Here's how the part is built. I have some questions about the finished solid (model axes, mm). A direction names the side the tool comes from. Give positions to 0.01 mm unless a question says otherwise; leave off trailing zeros. Write each loop counter-clockwise with the first axis right and the second up, starting at its lowest first coordinate (ties: lowest second). Pieces come first, ordered by that corner, then holes. Notation, with made-up numbers: (20, 5) -> (43, 5) arc R19 cw to (43, 13) -> close; hole circle Ø9 at (-12, -23). An arc over 180 degrees is marked (long way). Put each result on its own line as item: value. Start each with the question number.
from build123d import *

# Parameters (mm, degrees)
SKETCH1_W                    = 288.2
SKETCH1_H                    = 200
SKETCH1_R                    = 5
BASE_FLANGE1_DEPTH           = 3.4
EDGE_FLANGE2_STRIP_W         = 15.0732
EDGE_FLANGE2_STRIP_H         = 3.4
EDGE_FLANGE2_STRIP_CUT_DEPTH = 200
EDGE_FLANGE2_DEPTH           = 200
EDGE_FLANGE2_PROFILE_W       = 200
EDGE_FLANGE2_PROFILE_H       = 39.2634
EDGE_FLANGE2_PROFILE_R       = 5
EDGE_FLANGE2_FLAT_DEPTH      = 3.4
EDGE_FLANGE3_STRIP_W         = 15.0732
EDGE_FLANGE3_STRIP_H         = 3.4
EDGE_FLANGE3_STRIP_CUT_DEPTH = 200
EDGE_FLANGE3_DEPTH           = 200
EDGE_FLANGE3_PROFILE_W       = 200
EDGE_FLANGE3_PROFILE_H       = 39.2634
EDGE_FLANGE3_PROFILE_R       = 5
EDGE_FLANGE3_FLAT_DEPTH      = 3.4


# Sheet-metal steps are written as plain solids
with BuildPart() as part:
    # Sketch1 → Base-Flange1 (new body)
    with BuildSketch(Plane.XY):
        with Locations((-144.1, -100)):
            Rectangle(SKETCH1_W, SKETCH1_H)
        with Locations((-111.6, -100)):
            Circle(SKETCH1_R, mode=Mode.SUBTRACT)
        with Locations(Location((-176.6, -100, 0), (0, 0, 180))):
            Circle(SKETCH1_R, mode=Mode.SUBTRACT)
    extrude(amount=-BASE_FLANGE1_DEPTH)

    # Edge-Flange2 strip (across the edge) → Edge-Flange2 strip cut (cut)
    with BuildSketch(Plane(origin=(0, 0, -3.4), x_dir=(-1, 0, 0), z_dir=(0, -1, 0))):
        with Locations((-3.4, -1.7)):
            Rectangle(EDGE_FLANGE2_STRIP_W, EDGE_FLANGE2_STRIP_H)
    extrude(amount=EDGE_FLANGE2_STRIP_CUT_DEPTH, mode=Mode.SUBTRACT)

    # Edge-Flange2 bend section (across the edge) → Edge-Flange2 (add)
    with BuildSketch(Plane(origin=(0, 0, -3.4), x_dir=(-1, 0, 0), z_dir=(0, -1, 0))):
        with BuildLine():
            Line((0, 0.7366), (3.4, 0.7366))
            ThreePointArc((3.4, 0.7366), (3.615745145, 0.215745145), (4.1366, 0))
            Line((4.1366, 0), (4.1366, -3.4))
            ThreePointArc((4.1366, -3.4), (1.211582089, -2.188417911), (0, 0.7366))
        make_face()
    extrude(amount=EDGE_FLANGE2_DEPTH)

    # Edge-Flange2 profile (on flange) → Edge-Flange2 flat (add)
    with BuildSketch(Plane(origin=(0, 0, -3.4), x_dir=(0, -1, 0), z_dir=(1, 0, 0))):
        with Locations((100, 20.3683)):
            Rectangle(EDGE_FLANGE2_PROFILE_W, EDGE_FLANGE2_PROFILE_H)
        with Locations((150, 15.6)):
            Circle(EDGE_FLANGE2_PROFILE_R, mode=Mode.SUBTRACT)
        with Locations((50, 15.6)):
            Circle(EDGE_FLANGE2_PROFILE_R, mode=Mode.SUBTRACT)
    extrude(amount=-EDGE_FLANGE2_FLAT_DEPTH)

    # Edge-Flange3 strip (across the edge) → Edge-Flange3 strip cut (cut)
    with BuildSketch(Plane(origin=(-288.2, -200, -3.4), x_dir=(1, 0, 0), z_dir=(0, 1, 0))):
        with Locations((-3.4, -1.7)):
            Rectangle(EDGE_FLANGE3_STRIP_W, EDGE_FLANGE3_STRIP_H)
    extrude(amount=EDGE_FLANGE3_STRIP_CUT_DEPTH, mode=Mode.SUBTRACT)

    # Edge-Flange3 bend section (across the edge) → Edge-Flange3 (add)
    with BuildSketch(Plane(origin=(-288.2, -200, -3.4), x_dir=(1, 0, 0), z_dir=(0, 1, 0))):
        with BuildLine():
            Line((0, 0.7366), (3.4, 0.7366))
            ThreePointArc((3.4, 0.7366), (3.615745145, 0.215745145), (4.1366, 0))
            Line((4.1366, 0), (4.1366, -3.4))
            ThreePointArc((4.1366, -3.4), (1.211582089, -2.188417911), (0, 0.7366))
        make_face()
    extrude(amount=EDGE_FLANGE3_DEPTH)

    # Edge-Flange3 profile (on flange) → Edge-Flange3 flat (add)
    with BuildSketch(Plane(origin=(-288.2, 0, -3.4), x_dir=(0, 1, 0), z_dir=(-1, 0, 0))):
        with Locations((-100, 20.3683)):
            Rectangle(EDGE_FLANGE3_PROFILE_W, EDGE_FLANGE3_PROFILE_H)
        with Locations((-50, 15.6)):
            Circle(EDGE_FLANGE3_PROFILE_R, mode=Mode.SUBTRACT)
        with Locations((-150, 15.6)):
            Circle(EDGE_FLANGE3_PROFILE_R, mode=Mode.SUBTRACT)
    extrude(amount=-EDGE_FLANGE3_FLAT_DEPTH)


solid = part.part
1) I need wall thicknesses on probe 1 along Y at (x, z) = (-285.95, -19); probe 2 along X at (y, z) = (-117.5, -15.5); probe 3 along Y at (x, z) = (-176.6, -1). Which ranges of each line are inside material? Lowest first, please.
2) I'm going to push a flat-ended pin straight in: pin 1 Ø10 at (x, y) = (-114.5, -174) entering from -Z. Where does the tip first touch, or does it pass through?
3) Which directions (+Z, -Z, +X, -X, +Y, -Y) give clear straight access to the entire face, cutting with the end or side of a thin tool? Please do faces 5 (the flat face through (-145, -200, -1)), 6 (the flat face through (-3.4, -99, -24)).
4) I want a section at A-A, the plane z = -7. Write out the boundary of the cut face in (x, y).
5) I want a section at B-B, the plane y = -50. Write out the boundary of the cut face in (x, z), and give its area (3 significant figures).
6) I want a section at D-D, the plane y = -164. Write out the boundary of the cut face in (x, z).
7) I want a section at C-C, the plane x = -111.6. Write out the boundary of the cut face in (y, z).
8) Thinking about a two-plate mould opening in X: for faces 1 (the flat face through (0, -99, -24)), 2 (the cylindrical face through (-116.595, -99.78, -1.676)), 3 (the flat face through (-284.8, -101, -24)), 4 (the cylindrical face through (-287, -54, -16)), which applies, released by +X, released by -X, zero draft, split by the parting line, or undercut?
Established:
1. probe 1: y = -200 to -155, -145 to -55, -45 to 0
1. probe 2: x = -288.2 to -284.8, -3.4 to 0
1. probe 3: y = -200 to -105, -95 to 0
2. pin 1: stops at z = -3.4
3. face 5: +Z, -Z, +X, -X, -Y
3. face 6: -Z, +Y, -Y
4. outline: (-288.2, -200) -> (-284.8, -200) -> (-284.8, 0) -> (-288.2, 0) -> close; (-3.4, -200) -> (0, -200) -> (0, 0) -> (-3.4, 0) -> close
5. outline: (-288.2, -43.4) -> (-284.8, -43.4) -> (-284.8, -24) -> (-288.2, -24) -> close; (-288.2, -14) -> (-284.8, -14) -> (-284.8, -4.14) arc R0.74 cw to (-284.06, -3.4) -> (-4.14, -3.4) arc R0.74 cw to (-3.4, -4.14) -> (-3.4, -14) -> (0, -14) -> (0, -4.14) arc R4.14 ccw to (-4.14, 0) -> (-284.06, 0) arc R4.14 ccw to (-288.2, -4.14) -> close; (-3.4, -43.4) -> (0, -43.4) -> (0, -24) -> (-3.4, -24) -> close
5. area: 1,180 mm2
6. outline: (-288.2, -43.4) -> (-284.8, -43.4) -> (-284.8, -4.14) arc R0.74 cw to (-284.06, -3.4) -> (-4.14, -3.4) arc R0.74 cw to (-3.4, -4.14) -> (-3.4, -43.4) -> (0, -43.4) -> (0, -4.14) arc R4.14 ccw to (-4.14, 0) -> (-284.06, 0) arc R4.14 ccw to (-288.2, -4.14) -> close
7. outline: (-200, -3.4) -> (-105, -3.4) -> (-105, 0) -> (-200, 0) -> close; (-95, -3.4) -> (0, -3.4) -> (0, 0) -> (-95, 0) -> close
8. face 1: released by +X
8. face 2: undercut
8. face 3: undercut
8. face 4: zero draft
